Answer from the drawing. Dimensions are ordinates in mm from the lowest x, y and z of the part. A direction names the side the tool comes from. Coordinates: 2 decimals unless noted, no trailing zeros. Order: outer loops, then holes, each group sorted by start corner. A loop starts at its lowest first (then second) coordinate and runs counter-clockwise, first axis right, second up.
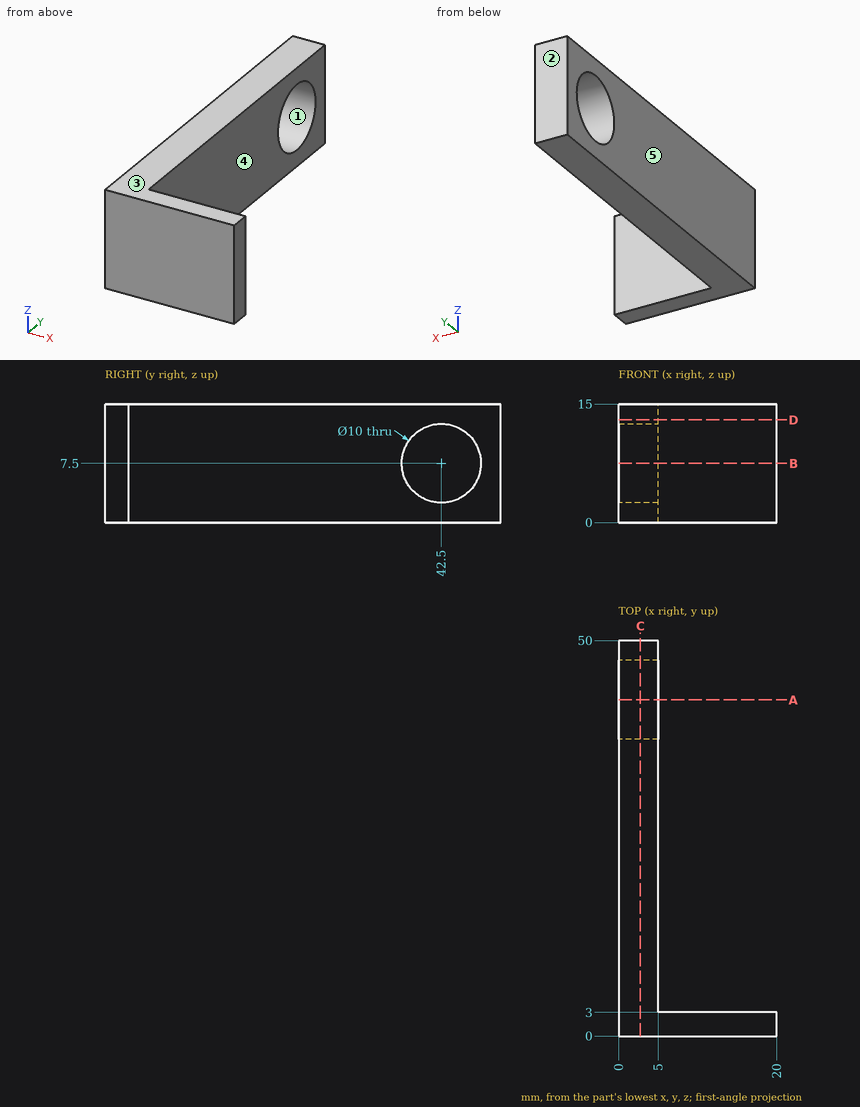
1. The part is cut by section B-B (z = 7.5). Determine the outline of the cut face in (x, y), plus the area to 3 significant figures.
2. Consider probe 1 along Y at (x, z) = (2.2, 7.5); probe 2 along X at (y, z) = (35.5, 12.5); probe 3 along Y at (x, z) = (13.5, 13.5). Determine where each line is inside the solid, lowest interval first.
3. For the marked faces 4 and 5, determine the directions among +Z, -Z, +X, -X, +Y, -Y from which every point of the face is accessible in a straight line to the end or side of a thin tool.
4. The part is cut by section C-C (x = 2.75). Determine the outline of the cut face in (y, z), plus the area to 3 significant figures.
5. The part is cut by section D-D (z = 13). Determine the outline of the cut face in (x, y).
6. The part is cut by section A-A (y = 42.5). Determine the outline of the cut face in (x, z), plus the area to 3 significant figures.
7. The mould has two halves that part along Z. Classify the marked faces 1, 2 and 3: released by +Z, released by -Z, zero draft, split by the parting line, or undercut.
8. Flat-ended cylindrical pins translate along their axes: pin 1 (8 mm diameter, centred on x = 5.5, z = 8.5, fed in from -Y); pin 2 (7.5 mm diameter, centred on y = 32.5, z = 11, fed in from +X); pin 3 (1.5 mm diameter, centred on x = 6, z = 11.5, fed in from +Y); pin 4 (9 mm diameter, centred on y = 42.5, z = 7.5, fed in from -X). Find the tip coordinate at first contact, or state that the pin passes through.
Worked out:
1. outline: (0, 0) - (20, 0) - (20, 3) - (5, 3) - (5, 37.5) - (0, 37.5) - close; (0, 47.5) - (5, 47.5) - (5, 50) - (0, 50) - close
1. area: 245 mm2
2. probe 1: y = 0 to 37.5, 47.5 to 50
2. probe 2: x = 0 to 5
2. probe 3: y = 0 to 3
3. face 4: +Z, -Z, +X, +Y
3. face 5: +Z, -Z, -X, +Y, -Y
4. outline: (0, 0) - (50, 0) - (50, 15) - (0, 15) - close; hole circle Ø10 at (42.5, 7.5)
4. area: 671 mm2
5. outline: (0, 0) - (20, 0) - (20, 3) - (5, 3) - (5, 50) - (0, 50) - close
6. outline: (0, 0) - (5, 0) - (5, 2.5) - (0, 2.5) - close; (0, 12.5) - (5, 12.5) - (5, 15) - (0, 15) - close
6. area: 25.0 mm2
7. face 1: undercut
7. face 2: zero draft
7. face 3: released by +Z
8. pin 1: stops at y = 0
8. pin 2: stops at x = 5
8. pin 3: stops at y = 3
8. pin 4: passes through
